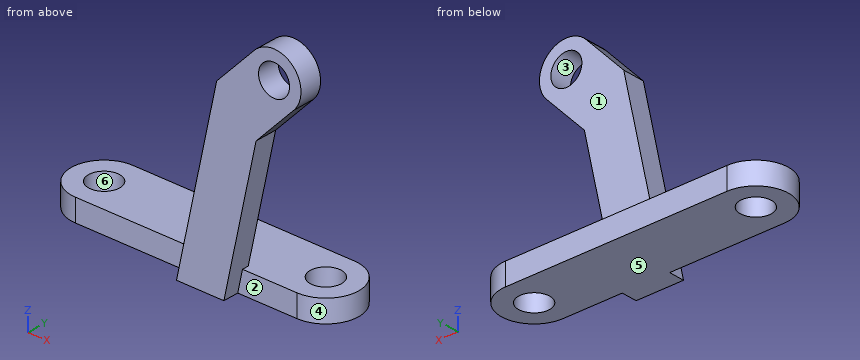
```python
from build123d import *

# Parameters (mm, degrees)
SKETCH1_R           = 1.75
BOSS_EXTRUDE1_DEPTH = 2.5
SKETCH2_R           = 1.75
BOSS_EXTRUDE2_DEPTH = 2.5


with BuildPart() as part:
    # Sketch1 → Boss-Extrude1 (new body)
    with BuildSketch(Plane.XY):
        with BuildLine():
            Line((-51.451246925, 1.046447779), (-76.451246925, 1.046447779))
            ThreePointArc((-76.451246925, 1.046447779), (-80.116799147, 4.712), (-76.451246925, 8.377552221))
            Line((-76.451246925, 8.377552221), (-51.451246925, 8.377552221))
            ThreePointArc((-51.451246925, 8.377552221), (-47.785694704, 4.712), (-51.451246925, 1.046447779))
        make_face()
        with Locations((-76.451246925, 4.712)):
            Circle(SKETCH1_R, mode=Mode.SUBTRACT)
        with Locations((-51.451246925, 4.712)):
            Circle(SKETCH1_R, mode=Mode.SUBTRACT)
    extrude(amount=BOSS_EXTRUDE1_DEPTH)

    # Sketch2 → Boss-Extrude2 (add)
    with BuildSketch(Plane.XZ.offset(-1.777778923)):
        with BuildLine():
            Line((-58.149633546, 0), (-54.518808092, 16.818393056))
            Line((-54.518808092, 16.818393056), (-50.271714816, 21.362782861))
            ThreePointArc((-50.271714816, 21.362782861), (-50.417137666, 25.663144264), (-54.717499069, 25.517721415))
            Line((-54.717499069, 25.517721415), (-58.964592345, 20.97333161))
            Line((-58.964592345, 20.97333161), (-63.492403415, 0))
            Line((-63.492403415, 0), (-58.149633546, 0))
        make_face()
        with Locations((-52.494606943, 23.440252138)):
            Circle(SKETCH2_R, mode=Mode.SUBTRACT)
    extrude(amount=BOSS_EXTRUDE2_DEPTH)


solid = part.part
```
For this review, take the finished solid that the model builds, in its own axes (mm). Face numbers are marked on the shaded views. A direction names the side the tool comes from. Round coordinates to 2 decimals unless told otherwise and drop trailing zeros. Write each loop counter-clockwise with the first axis right and the second up, starting at its lowest first coordinate (ties: lowest second). Pieces come first, ordered by that corner, then holes. Notation, with made-up numbers: (19, 11.5) - (58, 11.5) arc R22 cw to (58, 36.5) - close; hole circle Ø7 at (17, 69.25). An arc over 180 degrees is marked (long way). Use CSV: the item, a comma, the result in double quotes.
1) Clearance check with flat-ended pins moving along their axes: pin 1 Ø4 at (x, z) = (-59.5, 10) entering from +Y; pin 2 Ø2 at (x, z) = (-54.5, 1) entering from -Y; pin 3 Ø3 at (y, z) = (1, 20) entering from -X. State where each tip first meets the part, or that it passes through.
Conclusion:
pin 1,"stops at y = 1.78"
pin 2,"stops at y = 1.05"
pin 3,"stops at x = -59.5"
2) Add section C-C on x = -60.5. Write out the cut boundary in (y, z).
Conclusion:
outline,"(-0.72, 0) - (8.38, 0) - (8.38, 2.5) - (1.78, 2.5) - (1.78, 13.86) - (-0.72, 13.86) - close"
3) Add section B-B on y = 0.5. Write out the cut boundary in (x, z), and give its area (3 significant figures).
Conclusion:
outline,"(-63.49, 0) - (-58.15, 0) - (-54.52, 16.82) - (-50.27, 21.36) arc R3.04 ccw to (-54.72, 25.52) - (-58.96, 20.97) - close; hole circle Ø3.5 at (-52.49, 23.44)"
area,"144 mm^2"
4) Wall thickness on line 1 along Z through (x, y) = (-70, 3.5); line 2 along Y through (x, z) = (-56.5, 20); line 3 along Y through (x, z) = (-54.5, 2.25): over which ranges is each line inside the solid? List them lowest first. Write a range as from..to.
Conclusion:
line 1,"z = 0..2.5"
line 2,"y = -0.72..1.78"
line 3,"y = 1.05..8.38"
5) Add section D-D on z = 14.75. Write out the cut boundary in (x, y).
Conclusion:
outline,"(-60.31, -0.72) - (-54.97, -0.72) - (-54.97, 1.78) - (-60.31, 1.78) - close"
6) Add section A-A on y = 5.25. Write out the cut boundary in (x, z).
Conclusion:
outline,"(-80.08, 0) - (-78.12, 0) - (-78.12, 2.5) - (-80.08, 2.5) - close; (-74.79, 0) - (-53.12, 0) - (-53.12, 2.5) - (-74.79, 2.5) - close; (-49.79, 0) - (-47.83, 0) - (-47.83, 2.5) - (-49.79, 2.5) - close"
7) The part is to be moulded in two halves that separate along Y. For the marked faces 4, 5 and 6, say which applies: pulls with the +Y half, pulls with the -Y half, needs draft (parallel to the pull), parting line crosses it, or undercut.
Conclusion:
face 4,"parting line crosses it"
face 5,"needs draft"
face 6,"undercut"
8) For the marked faces 1, 2 and 3, list the 3-axis set-ups (+Z, -Z, +X, -X, +Y, -Y) from which the entire face can be reached by the end or side of a thin tool; tool diameter is ignored.
Conclusion:
face 1,"+Z, +X, -X, +Y"
face 2,"-Z, +X, -Y"
face 3,"+Y, -Y"
